Design review of the part built by this model. Coordinates are the model's own, in mm. A direction names the side the tool comes from. Give positions to 0.01 mm unless a question says otherwise; leave off trailing zeros. Write each loop counter-clockwise with the first axis right and the second up, starting at its lowest first coordinate (ties: lowest second). Pieces come first, ordered by that corner, then holes.
```python
from build123d import *

# Parameters (mm, degrees)
SKETCH1_R           = 59.41
SKETCH1_R_2         = 53.81
BOSS_EXTRUDE1_DEPTH = 10
SKETCH1_3_R         = 53.81
SKETCH1_3_R_2       = 30.2
SKETCH1_3_R_3       = 9.175
SKETCH1_3_R_4       = 24.69
BOSS_EXTRUDE2_DEPTH = 5
SKETCH1_4_R         = 30.2
SKETCH1_4_R_2       = 24.69
BOSS_EXTRUDE3_DEPTH = 8
SKETCH1_5_R         = 4.625
SKETCH1_5_R_2       = 9.175
CUT_EXTRUDE1_DEPTH  = 85.611442489
CIRPATTERN2_COUNT   = 8


with BuildPart() as part:
    # Sketch1 → Boss-Extrude1 (new, symmetric)
    with BuildSketch(Plane.XY):
        Circle(SKETCH1_R)
        Circle(SKETCH1_R_2, mode=Mode.SUBTRACT)
    extrude(amount=BOSS_EXTRUDE1_DEPTH, both=True)

    # Sketch1_3 → Boss-Extrude2 (add, symmetric)
    # profile 1 of 2: a face of its own
    with BuildSketch(Plane.XY):
        Circle(SKETCH1_3_R)
        Circle(SKETCH1_3_R_2, mode=Mode.SUBTRACT)
        with Locations((0, 43.035)):
            Circle(SKETCH1_3_R_3, mode=Mode.SUBTRACT)
    # profile 2 of 2: a face of its own
    with BuildSketch(Plane.XY):
        Circle(SKETCH1_3_R_4)
    extrude(amount=BOSS_EXTRUDE2_DEPTH, both=True)


with BuildPart() as boss_extrude2_piece_1:
    # of the separate pieces the step leaves, piece 1, a body of its own (boss_extrude2_pieces)
    add(part.part.solids().sort_by_distance((59.41, 0, -10))[0])



with BuildPart() as boss_extrude2_piece_2:
    # of the separate pieces the step leaves, piece 2, a body of its own (boss_extrude2_pieces)
    add(part.part.solids().sort_by_distance((24.69, 0, -5))[0])


with BuildPart() as boss_extrude2_piece_1_1:
    add(boss_extrude2_piece_1.part)

    add(boss_extrude2_piece_2.part)  # Boss-Extrude3 merges Boss-Extrude2 piece 2
    # Sketch1_4 → Boss-Extrude3 (add, symmetric)
    with BuildSketch(Plane.XY):
        Circle(SKETCH1_4_R)
        Circle(SKETCH1_4_R_2, mode=Mode.SUBTRACT)
    extrude(amount=BOSS_EXTRUDE3_DEPTH, both=True)

    # Sketch1_5 → Cut-Extrude1 (cut, symmetric)
    with BuildSketch(Plane.XY):
        with Locations((0, 17.024057501)):
            Circle(SKETCH1_5_R)
        with Locations((0, 43.035)):
            Circle(SKETCH1_5_R_2)
    cut_extrude1 = extrude(amount=CUT_EXTRUDE1_DEPTH, both=True, mode=Mode.SUBTRACT)

    # CirPattern2: Cut-Extrude1 ×8 about axis
    cirpattern2_axis = Axis((0, 0, 0), (0, 0, 1))
    for i in range(1, CIRPATTERN2_COUNT):
        add(cut_extrude1.rotate(cirpattern2_axis, i * 360 / CIRPATTERN2_COUNT), mode=Mode.SUBTRACT)


solid = boss_extrude2_piece_1_1.part
```
(1) Clearance check with flat-ended pins moving along their axes: P1, Ø4, axis at y = 23, z = 4, coming from the +X side; P2, Ø1.5, axis at x = 13.5, z = -3, coming from the +Y side; P3, Ø1.5, axis at x = 31, y = 10.5, coming from the +Z side. State where each tip first meets the part, or that it passes through.
Resolved:
P1: stops at x = 55.57
P2: stops at y = 58.03
P3: stops at z = 5
(2) Consider section B-B, the plane x = 0. Give the number of separate pieces and of enclosed holes in the cut face, then the cut area to 3 significant figures.
Resolved:
separate pieces: 5
enclosed holes: 0
area: 814 mm2
(3) Mouldability with a two-part tool opening along X and no side actions: class faces 1 (the face through (-12.879, -57.997, 0.14)), 2 (the face through (-31.1, 44.3, -10)), 3 (the face through (33.939, 21.953, 0.07)), 4 (the face through (-3.21, 24.48, -6.52)) as pulls with the +X half, pulls with the -X half, needs draft (parallel to the pull), parting line crosses it, or undercut.
Resolved:
face 1: parting line crosses it
face 2: needs draft
face 3: undercut
face 4: undercut
(4) To check wall thickness, follow L1, parallel to Y at x = 0, z = 2.3; L2, parallel to X at y = -22, z = 3.5; L3, parallel to Y at x = 33, z = -1. State the ranges of each line that lie inside material, in increasing order.
Resolved:
L1: y = -59.41 to -52.21, -33.86 to -21.65, -12.4 to 12.4, 21.65 to 33.86, 52.21 to 59.41
L2: x = -55.19 to -34.05, -26.81 to 26.81, 34.05 to 55.19
L3: y = -49.4 to -39.24, -21.62 to 21.62, 39.24 to 49.4
(5) Consider section A-A, the plane y = -46. Give the boundary of the cut face in (x, z).
Resolved:
outline: (-37.6, -10) - (-27.92, -10) - (-27.92, -5) - (-8.68, -5) - (-8.68, 5) - (-27.92, 5) - (-27.92, 10) - (-37.6, 10) - close; (8.68, -5) - (27.92, -5) - (27.92, -10) - (37.6, -10) - (37.6, 10) - (27.92, 10) - (27.92, 5) - (8.68, 5) - close
(6) Tool access review of faces 5 (the face through (0, 0, 5)), 6 (the face through (-33.939, -21.953, 0.07)), 7 (the face through (-12, 28, -5)): name each direction out of +Z, -Z, +X, -X, +Y, -Y from which nothing blocks a thin tool from reaching the whole face with its end or side.
Resolved:
face 5: +Z
face 6: +Z, -Z
face 7: -Z
(7) Consider section C-C, the plane y = -26.5. Give the boundary of the cut face in (x, z), then the cut area to 3 significant figures.
Resolved:
outline: (-53.17, -10) - (-46.83, -10) - (-46.83, -5) - (-38.72, -5) - (-38.72, 5) - (-46.83, 5) - (-46.83, 10) - (-53.17, 10) - close; (-22.14, -5) - (-14.48, -5) - (-14.48, -8) - (14.48, -8) - (14.48, -5) - (22.14, -5) - (22.14, 5) - (14.48, 5) - (14.48, 8) - (-14.48, 8) - (-14.48, 5) - (-22.14, 5) - close; (38.72, -5) - (46.83, -5) - (46.83, -10) - (53.17, -10) - (53.17, 10) - (46.83, 10) - (46.83, 5) - (38.72, 5) - close
area: 1,030 mm2
